```python
from build123d import *

# Parameters (mm, degrees)
SKETCH1_W           = 140
SKETCH1_H           = 140
BOSS_EXTRUDE1_DEPTH = 2
BOSS_EXTRUDE3_DEPTH = 2
FILLET1_R           = 10
SKETCH4_R           = 1.5
CUT_EXTRUDE2_DEPTH  = 2
SKETCH5_R           = 2.25
CUT_EXTRUDE3_DEPTH  = 10
SKETCH6_R           = 1.25
CUT_EXTRUDE4_DEPTH  = 15
CUT_EXTRUDE5_DEPTH  = 2


with BuildPart() as part:
    # Sketch1 → Boss-Extrude1 (new body)
    with BuildSketch(Plane(origin=(0, 0, 0), x_dir=(1, 0, 0), z_dir=(0, 1, 0))):
        with Locations((70, 70)):
            Rectangle(SKETCH1_W, SKETCH1_H)
    extrude(amount=BOSS_EXTRUDE1_DEPTH)

    # Sketch2 → Boss-Extrude3 (add)
    with BuildSketch(Plane(origin=(0, 2, 0), x_dir=(1, 0, 0), z_dir=(0, 1, 0))):
        Polygon((111.715728753, 140), (140, 111.715728753), (154.142135624, 125.857864376), (125.857864376, 154.142135624), align=None)
        Polygon((0, 111.715728753), (-14.142135624, 125.857864376), (14.142135624, 154.142135624), (28.284271247, 140), align=None)
        Polygon((28.284271247, 0), (0, 28.284271247), (-14.142135624, 14.142135624), (14.142135624, -14.142135624), align=None)
        Polygon((140, 28.284271247), (154.142135624, 14.142135624), (125.857864376, -14.142135624), (111.715728753, 0), align=None)
    extrude(amount=-BOSS_EXTRUDE3_DEPTH)

    # Fillet1
    fillet1_edges = [part.edges().sort_by_distance(p)[0] for p in [
        (125.857864376, 1, -154.142135624),
        (154.142135624, 1, -125.857864376),
        (-14.142135624, 1, -125.857864376),
        (14.142135624, 1, -154.142135624),
        (14.142135624, 1, 14.142135624),
        (-14.142135624, 1, -14.142135624),
        (154.142135624, 1, -14.142135624),
        (125.857864376, 1, 14.142135624),
    ]]
    fillet(fillet1_edges, radius=FILLET1_R)

    # Sketch4 → Cut-Extrude2 (cut)
    with BuildSketch(Plane(origin=(0, 2, 0), x_dir=(1, 0, 0), z_dir=(0, 1, 0))):
        with Locations(Location((38.717631804, 10.433360556, 0), (0, 0, 270))):
            Circle(SKETCH4_R)
        with Locations(Location((10.433360556, 38.717631804, 0), (0, 0, 90))):
            Circle(SKETCH4_R)
        with Locations(Location((101.282368196, 10.433360556, 0), (0, 0, 90))):
            Circle(SKETCH4_R)
        with Locations(Location((129.566639444, 38.717631804, 0), (0, 0, 270))):
            Circle(SKETCH4_R)
        with Locations(Location((38.717631804, 129.566639444, 0), (0, 0, 90))):
            Circle(SKETCH4_R)
        with Locations(Location((10.433360556, 101.282368196, 0), (0, 0, 270))):
            Circle(SKETCH4_R)
        with Locations(Location((101.282368196, 129.566639444, 0), (0, 0, 270))):
            Circle(SKETCH4_R)
        with Locations(Location((129.566639444, 101.282368196, 0), (0, 0, 90))):
            Circle(SKETCH4_R)
    extrude(amount=-CUT_EXTRUDE2_DEPTH, mode=Mode.SUBTRACT)

    # Sketch5 → Cut-Extrude3 (cut)
    with BuildSketch(Plane(origin=(0, 2, 0), x_dir=(1, 0, 0), z_dir=(0, 1, 0))):
        with Locations(Location((14.142135624, 14.142135624, 0), (0, 0, 270))):
            Circle(SKETCH5_R)
        with Locations(Location((125.857864376, 14.142135624, 0), (0, 0, 90))):
            Circle(SKETCH5_R)
        with Locations(Location((14.142135624, 125.857864376, 0), (0, 0, 90))):
            Circle(SKETCH5_R)
        with Locations(Location((125.857864376, 125.857864376, 0), (0, 0, 270))):
            Circle(SKETCH5_R)
    extrude(amount=-CUT_EXTRUDE3_DEPTH, mode=Mode.SUBTRACT)

    # Sketch6 → Cut-Extrude4 (cut)
    with BuildSketch(Plane(origin=(0, 2, 0), x_dir=(1, 0, 0), z_dir=(0, 1, 0))):
        with Locations(Location((90, 111.999971357, 0), (0, 0, 270))):
            Circle(SKETCH6_R)
        with Locations(Location((98, 41.999971357, 0), (0, 0, 270))):
            Circle(SKETCH6_R)
        with Locations(Location((42, 41.999971357, 0), (0, 0, 90))):
            Circle(SKETCH6_R)
        with Locations(Location((50, 111.999971357, 0), (0, 0, 90))):
            Circle(SKETCH6_R)
    extrude(amount=-CUT_EXTRUDE4_DEPTH, mode=Mode.SUBTRACT)

    # Sketch7 → Cut-Extrude5 (cut)
    with BuildSketch(Plane(origin=(0, 2, 0), x_dir=(1, 0, 0), z_dir=(0, 1, 0))):
        Polygon((75, 15), (70, 5), (65, 15), (70, 10), align=None)
    extrude(amount=-CUT_EXTRUDE5_DEPTH, mode=Mode.SUBTRACT)


solid = part.part
```
The listing builds one solid part. Answer for the finished solid, in the listing's coordinates (mm). A direction names the side the tool comes from. Coordinates: 2 decimals unless noted, no trailing zeros. Order: outer loops, then holes, each group sorted by start corner. A loop starts at its lowest first (then second) coordinate and runs counter-clockwise, first axis right, second up. Notation, with made-up numbers: M -10.75,79 L 28.25,79 A26 ccw 28.25,97 Z; hole C 64,85 d6. An arc over 180 degrees is marked long. Answer as a JSON object with one key per item and string values. Group by question number.
1. Section A-A on x = 2.5 is taken. Write down the section's boundary in (y, z).
2. Section B-B on y = 0.4 is taken. State how many separate pieces and enclosed holes the cut face has, then the cut area to 3 significant figures.
3. Section C-C on z = -106 is taken. Write down the section's boundary in (x, y), then the cut area to 3 significant figures.
4. Determine the mould class of faces 1 (the flat face through (67.535, 1.014, -9.93)), 2 (the flat face through (140, 1, -140)), 3 (the flat face through (69, 2, -71)), 4 (the flat face through (24.699, 1.014, -143.585)) for opening direction X: released by +X, released by -X, zero draft, split by the parting line, or undercut.
5. Straight lines are drawn through the part: line 1 (X direction, y = 0.6, z = -38.5); line 2 (Z direction, x = 125, y = 1.6); line 3 (Z direction, x = 90, y = 1.3). For each, find the intervals that lie inside material, in ascending order.
6. A tool of negligible diameter and unlimited length cuts with its end or side. For faces 5 (the flat face through (115.301, 1.014, 3.585)), 6 (the flat face through (-3.486, 1.014, -24.798)), 7 (the cylindrical face through (123.627, 1.014, -13.849)), 8 (the flat face through (143.486, 1.014, -24.798)), from which of +Z, -Z, +X, -X, +Y, -Y can it reach the whole face along a straight path? Write none if from no direction.
7. Flat-ended cylindrical pins translate along their axes: P1, Ø0.6, axis at x = 80, y = 1.5, coming from the -Z side; P2, Ø0.6, axis at y = 1, z = -74, coming from the -X side; P3, Ø0.6, axis at y = 1, z = -69, coming from the +X side. Find the tip coordinate at first contact, or state that the pin passes through.
Values follow:
{
 "1": {"outline": "M 0,-142.5 L 2,-142.5 L 2,2.5 L 0,2.5 Z"},
 "2": {"separate pieces": "1", "enclosed holes": "17", "area": "20,900 mm2"},
 "3": {"outline": "M 0,0 L 140,0 L 140,2 L 0,2 Z", "area": "280 mm2"},
 "4": {"face 1": "undercut", "face 2": "released by +X", "face 3": "zero draft", "face 4": "undercut"},
 "5": {"line 1": "0 to 8.95, 11.92 to 128.08, 131.05 to 140", "line 2": "-149.96 to -127.94, -123.78 to -16.22, -12.06 to 9.96", "line 3": "-140 to -113.25, -110.75 to 0"},
 "6": {"face 5": "+Z, +Y, -Y", "face 6": "-X, +Y, -Y", "face 7": "+Y, -Y", "face 8": "+X, +Y, -Y"},
 "7": {"P1": "z = -140", "P2": "x = 0", "P3": "x = 140"}
}
